Design review of the part built by this model. Coordinates are the model's own, in mm. A direction names the side the tool comes from. Coordinates: 2 decimals unless noted, no trailing zeros. Loops run counter-clockwise (first coordinate to the right, second up) from the corner with the lowest first, then second, coordinate; pieces in that order, holes last. Notation, with made-up numbers: (88, -27.75) - (129, -27.75) arc R29 cw to (129, -3.75) - close; hole circle Ø6 at (33.25, 20). An arc over 180 degrees is marked (long way). Answer in a Markdown table with one row per item. Add a question column.
(1) For faces 1 (the face through (-25.945, 13.326, -0.111)), 2 (the face through (-4, 15.88, -4)), 3 (the face through (-17.4, 33.3, -20)), list the 3-axis set-ups (+Z, -Z, +X, -X, +Y, -Y) from which the entire face can be reached by the end or side of a thin tool; tool diameter is ignored.
(2) To check wall thickness, follow L1, parallel to X at y = 19.5, z = -4.5; L2, parallel to Y at x = -13, z = -6.5; L3, parallel to X at y = 6, z = -17.5. State the ranges of each line that lie inside material, in increasing order. Write a range as [from, to].
(3) We need section D-D, the plane y = 9.5. Write out the cut boundary in (x, z), plus the area to 3 significant figures.
(4) The part is to be moulded in two halves that separate along Y. For faces 4 (the face through (-35.9, 10.7, -16.3)), 5 (the face through (-3.45, 20.74, -5.64)), 6 (the face through (-17, 10.7, -18)), say which applies: released by +Y, released by -Y, zero draft, split by the parting line, or undercut.
(5) We need section A-A, the plane y = 20.5. Write out the cut boundary in (x, z).
(6) We need section C-C, the plane x = -4.5. Write out the cut boundary in (y, z).
(7) Clearance check with flat-ended pins moving along their axes: pin 1 (4 mm diameter, centred on y = 22, z = -23.5, fed in from -X); pin 2 (2 mm diameter, centred on y = 27, z = -19, fed in from +X); pin 3 (1.5 mm diameter, centred on y = 36, z = -18.5, fed in from -X). State where each tip first meets the part, or that it passes through.
from build123d import *

# Parameters (mm, degrees)
SKETCH1_R           = 4.5
BOSS_EXTRUDE1_DEPTH = 10.7
BOSS_EXTRUDE2_DEPTH = 5.18
BOSS_EXTRUDE3_DEPTH = 8.66
SKETCH5_R           = 1.55
CUT_EXTRUDE1_DEPTH  = 7.5
SKETCH6_R           = 11
BOSS_EXTRUDE4_DEPTH = 2
SKETCH7_R           = 2.5
BOSS_EXTRUDE5_DEPTH = 14.2
CHAMFER1_SIZE       = 0.2
FILLET1_R           = 0.5
FILLET2_R           = 0.7
CHAMFER2_SIZE       = 0.5
FILLET3_R           = 1.5


with BuildPart() as part:
    # Sketch1 → Boss-Extrude1 (new body)
    with BuildSketch(Plane(origin=(0, 0, 0), x_dir=(1, 0, 0), z_dir=(0, 1, 0))):
        Polygon((-35, 32.5), (-32.5, 35), (-2.5, 35), (0, 32.5), (0, 2.5), (-2.5, 0), (-32.5, 0), (-35, 2.5), (-35, 6.85), (-36.65, 6.85), (-36.65, 28.15), (-35, 28.15), align=None)
        with Locations(Location((-17.5, 17.5, 0), (0, 0, 270))):
            Circle(SKETCH1_R, mode=Mode.SUBTRACT)
    extrude(amount=BOSS_EXTRUDE1_DEPTH)

    # Sketch2 → Boss-Extrude2 (add)
    with BuildSketch(Plane(origin=(0, 10.7, 0), x_dir=(1, 0, 0), z_dir=(0, 1, 0))):
        Polygon((-26, 35), (-9, 35), (0, 26), (0, 9), (-9, 0), (-26, 0), (-35, 9), (-35, 26), align=None)
    extrude(amount=BOSS_EXTRUDE2_DEPTH)

    # Sketch3 → Boss-Extrude3 (add)
    with BuildSketch(Plane(origin=(0, 15.88, 0), x_dir=(1, 0, 0), z_dir=(0, 1, 0))):
        Polygon((-35, 2.5), (-35, 32.5), (-32.5, 35), (-2.5, 35), (0, 32.5), (0, 2.5), (-2.5, 0), (-32.5, 0), align=None)
    extrude(amount=BOSS_EXTRUDE3_DEPTH)

    # Sketch5 → Cut-Extrude1 (cut)
    with BuildSketch(Plane(origin=(0, 24.54, 0), x_dir=(1, 0, 0), z_dir=(0, 1, 0))):
        with Locations(Location((-30.5, 4.5, 0), (0, 0, 270))):
            Circle(SKETCH5_R)
        with Locations(Location((-4.5, 30.5, 0), (0, 0, 270))):
            Circle(SKETCH5_R)
        with Locations(Location((-30.5, 30.5, 0), (0, 0, 270))):
            Circle(SKETCH5_R)
        with Locations(Location((-4.5, 4.5, 0), (0, 0, 270))):
            Circle(SKETCH5_R)
    extrude(amount=-CUT_EXTRUDE1_DEPTH, mode=Mode.SUBTRACT)

    # Sketch6 → Boss-Extrude4 (add)
    with BuildSketch(Plane(origin=(0, 24.54, 0), x_dir=(1, 0, 0), z_dir=(0, 1, 0))):
        with Locations(Location((-17.5, 17.5, 0), (0, 0, 270))):
            Circle(SKETCH6_R)
    extrude(amount=BOSS_EXTRUDE4_DEPTH)

    # Sketch7 → Boss-Extrude5 (add)
    with BuildSketch(Plane(origin=(0, 26.54, 0), x_dir=(1, 0, 0), z_dir=(0, 1, 0))):
        with Locations(Location((-17.5, 17.5, 0), (0, 0, 270))):
            Circle(SKETCH7_R)
    extrude(amount=BOSS_EXTRUDE5_DEPTH)

    # Chamfer1
    chamfer1_edges = [part.edges().sort_by_distance(p)[0] for p in [
        (-4.5, 24.54, -6.05),
        (-30.5, 24.54, -32.05),
        (-4.5, 24.54, -32.05),
        (-30.5, 24.54, -6.05),
    ]]
    chamfer(chamfer1_edges, length=CHAMFER1_SIZE)

    # Fillet1
    fillet1_edges = [part.edges().sort_by_distance(p)[0] for p in [
        (-36.65, 5.35, -28.15),
        (-36.65, 10.7, -17.5),
        (-36.65, 5.35, -6.85),
        (-17.5, 0, -22),
        (-35.825, 0, -28.15),
        (-36.65, 0, -17.5),
        (-35.825, 0, -6.85),
        (-35, 0, -4.675),
        (-33.75, 0, -1.25),
        (-17.5, 0, 0),
        (-1.25, 0, -1.25),
        (0, 0, -17.5),
        (-1.25, 0, -33.75),
        (-17.5, 0, -35),
        (-33.75, 0, -33.75),
        (-2.5, 5.35, -35),
        (0, 5.35, -32.5),
        (-32.5, 5.35, -35),
        (0, 5.35, -2.5),
        (-2.5, 5.35, 0),
        (-32.5, 5.35, 0),
        (-35, 5.35, -2.5),
        (-35, 20.21, -32.5),
        (-33.75, 24.54, -33.75),
        (-32.5, 20.21, -35),
        (-17.5, 24.54, -35),
        (-2.5, 20.21, -35),
        (0, 20.21, -32.5),
        (0, 24.54, -17.5),
        (-1.25, 24.54, -33.75),
        (0, 20.21, -2.5),
        (-2.5, 20.21, 0),
        (-35, 20.21, -2.5),
        (-32.5, 20.21, 0),
        (-1.25, 24.54, -1.25),
        (-17.5, 24.54, 0),
        (-33.75, 24.54, -1.25),
        (-35, 24.54, -17.5),
        (-35, 0, -30.325),
    ]]
    fillet(fillet1_edges, radius=FILLET1_R)

    # Fillet2
    fillet2_edges = [part.edges().sort_by_distance(p)[0] for p in [
        (-17.5, 24.54, -28.5),
    ]]
    fillet(fillet2_edges, radius=FILLET2_R)

    # Chamfer2
    chamfer2_edges = [part.edges().sort_by_distance(p)[0] for p in [
        (-17.5, 40.74, -20),
    ]]
    chamfer(chamfer2_edges, length=CHAMFER2_SIZE)

    # Fillet3
    fillet3_edges = [part.edges().sort_by_distance(p)[0] for p in [
        (-26, 13.29, -35),
        (-35, 13.29, -26),
        (-35, 13.29, -9),
        (-26, 13.29, 0),
        (-9, 13.29, 0),
        (0, 13.29, -9),
        (0, 13.29, -26),
        (-9, 13.29, -35),
    ]]
    fillet(fillet3_edges, radius=FILLET3_R)


solid = part.part
Responses:
| question | item | result |
|---|---|---|
| 1 | face 1 | +Z, -X |
| 1 | face 2 | +Z, +X |
| 1 | face 3 | +Y |
| 2 | L1 | x = [-35, -32.05], [-28.95, -6.05], [-2.95, 0] |
| 2 | L2 | y = [0, 24.54] |
| 2 | L3 | x = [-36.65, -22], [-13, 0] |
| 3 | outline | (-36.65, -27.65) arc R0.5 ccw to (-36.15, -28.15) - (-35, -28.15) - (-35, -32.5) - (-32.65, -34.85) arc R0.5 ccw to (-32.29, -35) - (-2.71, -35) arc R0.5 ccw to (-2.35, -34.85) - (-0.15, -32.65) arc R0.5 ccw to (0, -32.29) - (0, -2.71) arc R0.5 ccw to (-0.15, -2.35) - (-2.35, -0.15) arc R0.5 ccw to (-2.71, 0) - (-32.29, 0) arc R0.5 ccw to (-32.65, -0.15) - (-34.85, -2.35) arc R0.5 ccw to (-35, -2.71) - (-35, -6.85) - (-36.15, -6.85) arc R0.5 ccw to (-36.65, -7.35) - close; hole circle Ø9 at (-17.5, -17.5) |
| 3 | area | 1,180 mm2 |
| 4 | face 4 | undercut |
| 4 | face 5 | zero draft |
| 4 | face 6 | released by -Y |
| 5 | outline | (-35, -32.29) arc R0.5 ccw to (-34.85, -32.65) - (-32.65, -34.85) arc R0.5 ccw to (-32.29, -35) - (-2.71, -35) arc R0.5 ccw to (-2.35, -34.85) - (-0.15, -32.65) arc R0.5 ccw to (0, -32.29) - (0, -2.71) arc R0.5 ccw to (-0.15, -2.35) - (-2.35, -0.15) arc R0.5 ccw to (-2.71, 0) - (-32.29, 0) arc R0.5 ccw to (-32.65, -0.15) - (-34.85, -2.35) arc R0.5 ccw to (-35, -2.71) - close; hole circle Ø3.1 at (-30.5, -30.5); hole circle Ø3.1 at (-30.5, -4.5); hole circle Ø3.1 at (-4.5, -30.5); hole circle Ø3.1 at (-4.5, -4.5) |
| 6 | outline | (0, -34.5) arc R0.5 ccw to (0.5, -35) - (10.7, -35) - (10.7, -30.5) - (15.88, -30.5) - (15.88, -35) - (24.04, -35) arc R0.5 ccw to (24.54, -34.5) - (24.54, -32.25) - (24.34, -32.05) - (17.04, -32.05) - (17.04, -28.95) - (24.34, -28.95) - (24.54, -28.75) - (24.54, -6.25) - (24.34, -6.05) - (17.04, -6.05) - (17.04, -2.95) - (24.34, -2.95) - (24.54, -2.75) - (24.54, -0.5) arc R0.5 ccw to (24.04, 0) - (15.88, 0) - (15.88, -4.5) - (10.7, -4.5) - (10.7, 0) - (0.5, 0) arc R0.5 ccw to (0, -0.5) - close |
| 7 | pin 1 | stops at x = -35 |
| 7 | pin 2 | stops at x = -6.52 |
| 7 | pin 3 | stops at x = -19.99 |
